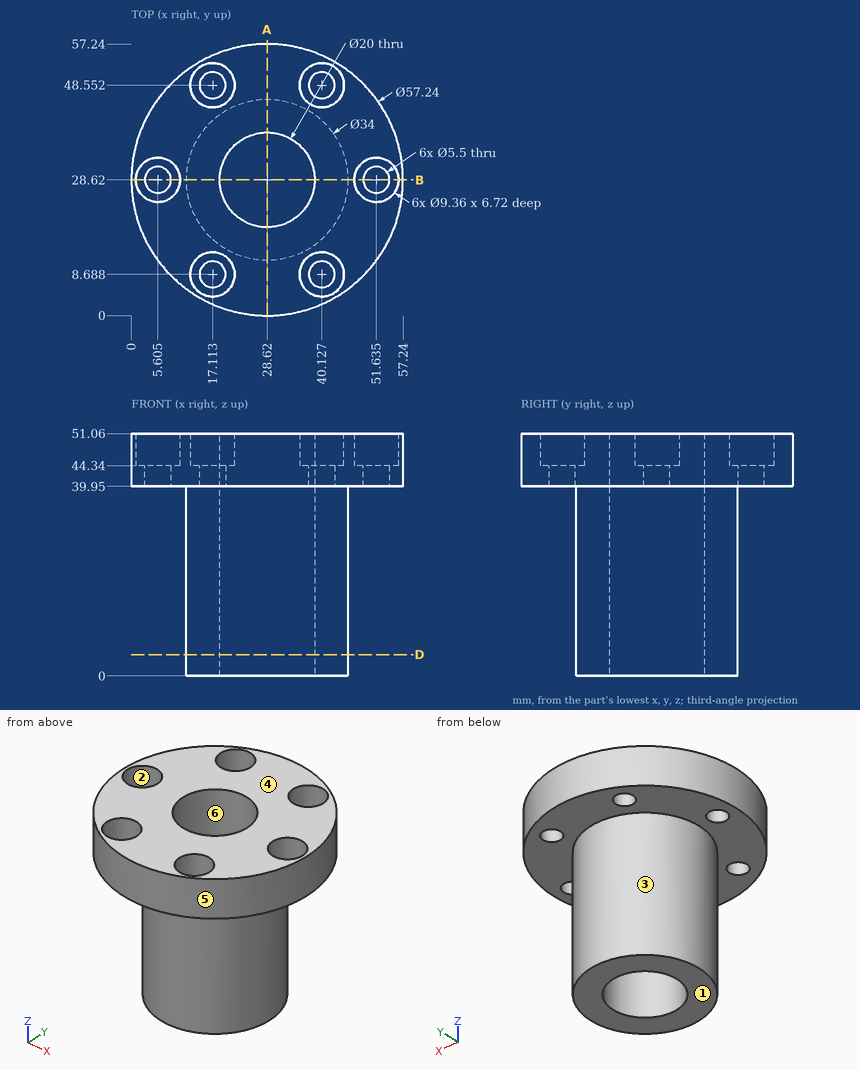
Design review of the part shown in the three views and the two pictorial views. Dimensions are in mm from the part's minimum x, y and z. A direction names the side the tool comes from. Coordinates: 2 decimals unless noted, no trailing zeros. Write each loop counter-clockwise with the first axis right and the second up, starting at its lowest first coordinate (ties: lowest second). Pieces come first, ordered by that corner, then holes.
(1) The part is to be moulded in two halves that separate along Y. For the marked faces 4, 5 and 6, say which applies: +Y half, -Y half, draft (parallel to the pull), parting line (faces both ways), or undercut.
(2) Wall thickness on probe 1 along Y at (x, z) = (40, 42) (1 decimal); probe 2 along X at (y, z) = (50.5, 46.5) (1 decimal); probe 3 along Z at (x, y) = (35.5, 53): over which ranges is each line inside the solid? List them lowest first.
(3) Add section B-B on y = 28.62. Count the separate pieces of the cut face and the enclosed holes in it, then the cut area to 3 significant figures.
(4) Tool access review of the marked faces 1, 2 and 3: name each direction out of +Z, -Z, +X, -X, +Y, -Y from which nothing blocks a thin tool from reaching the whole face with its end or side.
(5) Add section A-A on x = 28.62. Give the boundary of the cut face in (y, z), then the cut area to 3 significant figures.
(6) For pin 1 Ø7.5 at (x, y) = (52, 28) entering from +Z; pin 2 Ø7.5 at (x, y) = (51.635, 28.62) entering from -Z; pin 3 Ø6 at (y, z) = (10.5, 35.5) entering from -X; pin 4 Ø3.5 at (x, y) = (17.11, 48.55) entering from -Z, all flat-tipped, find the tip position at first contact; note any pin that passes through.
(7) Add section D-D on z = 4.5. Give the boundary of the cut face in (x, y), then the cut area to 3 significant figures.
Answer sheet:
1. face 4: draft
1. face 5: parting line
1. face 6: undercut
2. probe 1: y = 2.4 to 5.9, 11.4 to 45.8, 51.3 to 54.9
2. probe 2: x = 10.2 to 12.9, 21.4 to 35.9, 44.4 to 47.1
2. probe 3: z = 39.95 to 51.06
3. separate pieces: 4
3. enclosed holes: 0
3. area: 799 mm2
4. face 1: -Z, +X, -X, +Y, -Y
4. face 2: +Z
4. face 3: -Z
5. outline: (0, 39.95) - (11.62, 39.95) - (11.62, 0) - (18.62, 0) - (18.62, 51.06) - (0, 51.06) - close; (38.62, 0) - (45.62, 0) - (45.62, 39.95) - (57.24, 39.95) - (57.24, 51.06) - (38.62, 51.06) - close
5. area: 973 mm2
6. pin 1: stops at z = 44.34
6. pin 2: stops at z = 39.95
6. pin 3: stops at x = 20.85
6. pin 4: passes through
7. outline: circle Ø34 at (28.62, 28.62); hole circle Ø20 at (28.62, 28.62)
7. area: 594 mm2
